Here's the drawing with two shaded views (mm, measured from the low corner). I have some questions. A direction names the side the tool comes from. Give positions to 0.01 mm unless a question says otherwise; leave off trailing zeros. Write each loop counter-clockwise with the first axis right and the second up, starting at its lowest first coordinate (ties: lowest second). Pieces come first, ordered by that corner, then holes.
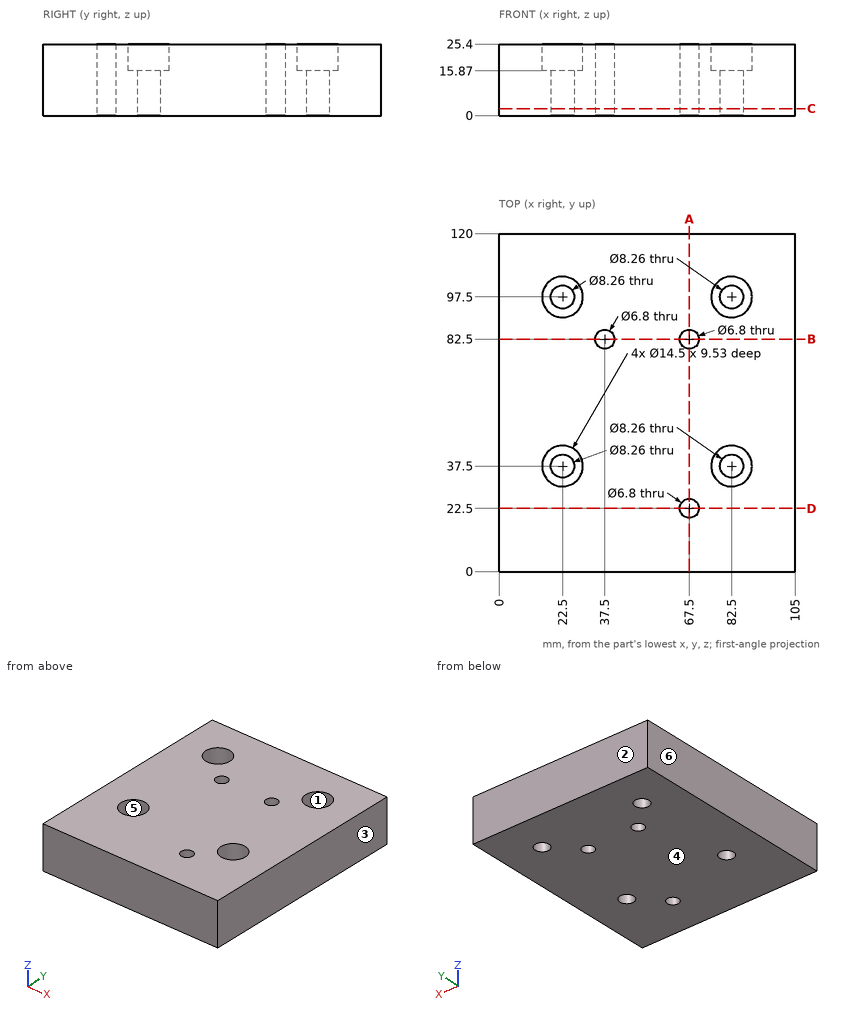
(1) Imagine slicing it at C-C, the plane z = 2.5. Write out the boundary of the cut face in (x, y), plus the area to 3 significant figures.
Returned:
outline: (0, 0) - (105, 0) - (105, 120) - (0, 120) - close; hole circle Ø8.26 at (22.5, 37.5); hole circle Ø8.26 at (22.5, 97.5); hole circle Ø6.8 at (37.5, 82.5); hole circle Ø6.8 at (67.5, 22.5); hole circle Ø6.8 at (67.5, 82.5); hole circle Ø8.26 at (82.5, 37.5); hole circle Ø8.26 at (82.5, 97.5)
area: 12,300 mm2
(2) If I drill on L1, parallel to Y at x = 67.5, z = 10.5; L2, parallel to Y at x = 22.5, z = 23.5; L3, parallel to X at y = 23, z = 23, over which ranges is the centre line in solid material (lowest first)?
Returned:
L1: y = 0 to 19.1, 25.9 to 79.1, 85.9 to 120
L2: y = 0 to 30.25, 44.75 to 90.25, 104.75 to 120
L3: x = 0 to 64.14, 70.86 to 105
(3) If we mould it in two halves opening along X, with no side actions, what happens to the marked faces 3, 4, 5 and 6? For each: +X half, -X half, draft (parallel to the pull), parting line (faces both ways), or undercut.
Returned:
face 3: +X half
face 4: draft
face 5: undercut
face 6: -X half
(4) Will this pin go through, and if not, where does the flat tip stop? P1, Ø7, axis at x = 21.5, y = 96.5, coming from the +Z side.
Returned:
P1: stops at z = 15.87
(5) Imagine slicing it at A-A, the plane x = 67.5. Write out the boundary of the cut face in (y, z).
Returned:
outline: (0, 0) - (19.1, 0) - (19.1, 25.4) - (0, 25.4) - close; (25.9, 0) - (79.1, 0) - (79.1, 25.4) - (25.9, 25.4) - close; (85.9, 0) - (120, 0) - (120, 25.4) - (85.9, 25.4) - close
(6) For the marked faces 1 and 2, which set-ups out of +Z, -Z, +X, -X, +Y, -Y let a thin tool reach every point of the face, with its end or its side?
Returned:
face 1: +Z
face 2: +Z, -Z, +X, -X, +Y
(7) Imagine slicing it at B-B, the plane y = 82.5. Write out the boundary of the cut face in (x, z), plus the area to 3 significant figures.
Returned:
outline: (0, 0) - (34.1, 0) - (34.1, 25.4) - (0, 25.4) - close; (40.9, 0) - (64.1, 0) - (64.1, 25.4) - (40.9, 25.4) - close; (70.9, 0) - (105, 0) - (105, 25.4) - (70.9, 25.4) - close
area: 2,320 mm2
(8) Imagine slicing it at D-D, the plane y = 22.5. Write out the boundary of the cut face in (x, z), plus the area to 3 significant figures.
Returned:
outline: (0, 0) - (64.1, 0) - (64.1, 25.4) - (0, 25.4) - close; (70.9, 0) - (105, 0) - (105, 25.4) - (70.9, 25.4) - close
area: 2,490 mm2
